Check sheet for the modelled part. Datum: model origin and axes. Units: mm. Face numbers are marked on the shaded views. A direction names the side the tool comes from. Give positions to 0.01 mm unless a question says otherwise; leave off trailing zeros. Order: outer loops, then holes, each group sorted by start corner. A loop starts at its lowest first (then second) coordinate and runs counter-clockwise, first axis right, second up.
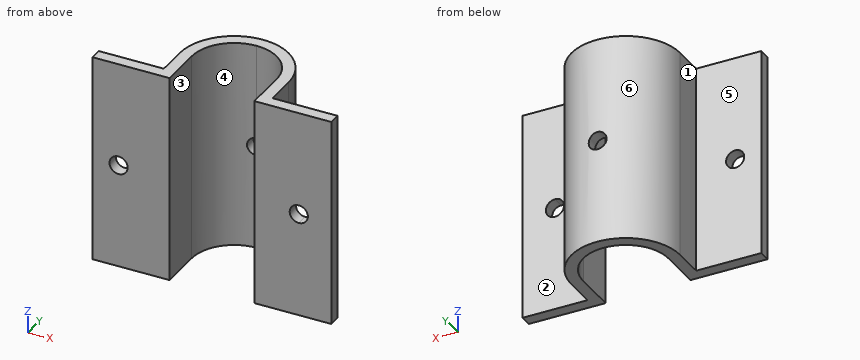
```python
from build123d import *

# Parameters (mm, degrees)
BOSS_EXTRUDE1_DEPTH = 70
SKETCH2_R           = 3.048
CUT_EXTRUDE1_DEPTH  = 70
FILLET1_R           = 14.224
FILLET2_RADIUS      = 18.224
FILLET2_LENGTH      = 70
SKETCH3_R           = 3
CUT_EXTRUDE2_DEPTH  = 70


with BuildPart() as part:
    # Sketch1 → Boss-Extrude1 (new body)
    with BuildSketch(Plane.XY):
        Polygon((-40.068, 0), (-18.224, 0), (-18.224, 28.448), (18.224, 28.448), (18.224, 0), (40.068, 0), (40.068, -4), (14.224, -4), (14.224, 24.448), (-14.224, 24.448), (-14.224, -4), (-40.068, -4), align=None)
    extrude(amount=BOSS_EXTRUDE1_DEPTH)

    # Sketch2 → Cut-Extrude1 (cut)
    with BuildSketch(Plane(origin=(0, 0, 0), x_dir=(1, 0, 0), z_dir=(0, 1, 0))):
        with Locations(Location((-31.280253866, -35, 0), (0, 0, 180))):
            Circle(SKETCH2_R)
        with BuildLine():
            ThreePointArc((32.194, -35), (31.301261469, -32.844738531), (29.146, -31.952))
            Line((29.146, -31.952), (29.146, -38.048))
            ThreePointArc((29.146, -38.048), (31.301261469, -37.155261469), (32.194, -35))
        make_face()
        with BuildLine():
            Line((29.146, -38.048), (29.146, -31.952))
            ThreePointArc((29.146, -31.952), (26.098, -35), (29.146, -38.048))
        make_face()
    extrude(amount=-CUT_EXTRUDE1_DEPTH, mode=Mode.SUBTRACT)

    # Fillet1
    fillet1_edges = [part.edges().sort_by_distance(p)[0] for p in [
        (14.224, 24.448, 35),
        (-14.224, 24.448, 35),
    ]]
    fillet(fillet1_edges, radius=FILLET1_R - 0.0001)  # a hair under: the kernel refuses the full size

    # Fillet2: full round fillet: the end face becomes a half cylinder, R = half its width
    fillet2_face = Plane((0, 28.448, 35), x_dir=(0, 0, 1), z_dir=(0, 1, 0))  # on the end face: x along it, z out of the body
    fillet2_slab = fillet2_face.offset(-FILLET2_RADIUS / 2) * Box(FILLET2_LENGTH, 2 * FILLET2_RADIUS, FILLET2_RADIUS, mode=Mode.PRIVATE)  # the body's end, R deep
    fillet2_round = Plane((0, 10.224, 35), x_dir=(0, 1, 0), z_dir=(0, 0, 1)) * Cylinder(FILLET2_RADIUS, FILLET2_LENGTH, mode=Mode.PRIVATE)  # its axis R under the face
    add(fillet2_slab - fillet2_round, mode=Mode.SUBTRACT)

    # Sketch3 → Cut-Extrude2 (cut)
    with BuildSketch(Plane(origin=(0, 0, 0), x_dir=(1, 0, 0), z_dir=(0, 1, 0))):
        with Locations(Location((0, -35, 0), (0, 0, 90))):
            Circle(SKETCH3_R)
    extrude(amount=CUT_EXTRUDE2_DEPTH, mode=Mode.SUBTRACT)


solid = part.part
```
(1) Cross-section at C-C on z = 33.5. Enter the section's corners in (x, y), then the cut area to 3 significant figures.
Response values:
outline: (-40.07, -4) - (-33.93, -4) - (-33.93, 0) - (-40.07, 0) - close; (-28.63, -4) - (-14.22, -4) - (-14.22, 10.22) arc R14.22 cw to (-2.6, 24.21) - (-2.6, 28.26) arc R18.22 ccw to (-18.22, 10.22) - (-18.22, 0) - (-28.63, 0) - close; (2.6, 24.21) arc R14.22 cw to (14.22, 10.22) - (14.22, -4) - (26.49, -4) - (26.49, 0) - (18.22, 0) - (18.22, 10.22) arc R18.22 ccw to (2.6, 28.26) - close; (31.8, -4) - (40.07, -4) - (40.07, 0) - (31.8, 0) - close
area: 429 mm2
(2) Set-up check for the marked faces 1, 2 and 3: record each of +Z, -Z, +X, -X, +Y, -Y from which the full face is reachable in a straight line by a thin tool's end or side.
Response values:
face 1: +Z, -Z, -X, +Y
face 2: +Z, -Z, +X, +Y
face 3: +Z, -Z, -Y
(3) Gauge pin test, flat ends, axial feed: pin 1 Ø1.5 at (x, z) = (-10, 50.5) entering from -Y; pin 2 Ø8 at (y, z) = (10, 58.5) entering from -X; pin 3 Ø1 at (x, z) = (30.5, 19.5) entering from +Y. Record the tip position at first contact, or that the pin passes through.
Response values:
pin 1: stops at y = 19.54
pin 2: stops at x = -18.22
pin 3: stops at y = 0
(4) Material ranges on L1, parallel to X at y = 8, z = 48; L2, parallel to Y at x = -29, z = 53; L3, parallel to X at y = 17.5, z = 65, recorded low to high.
Response values:
L1: x = -18.22 to -14.22, 14.22 to 18.22
L2: y = -4 to 0
L3: x = -16.71 to -12.22, 12.22 to 16.71
(5) Cross-section at B-B on y = 8. Enter the section's corners in (x, z).
Response values:
outline: (-18.22, 0) - (-14.22, 0) - (-14.22, 70) - (-18.22, 70) - close; (14.22, 0) - (18.22, 0) - (18.22, 70) - (14.22, 70) - close
(6) Release check for a two-part mould opening along X. For the marked faces 4, 5 and 6 record: released by +X, released by -X, zero draft, split by the parting line, or undercut.
Response values:
face 4: undercut
face 5: zero draft
face 6: split by the parting line
(7) Cross-section at A-A on y = -1. Enter the section's corners in (x, z), then the cut area to 3 significant figures.
Response values:
outline: (-40.07, 0) - (-14.22, 0) - (-14.22, 70) - (-40.07, 70) - close; (14.22, 0) - (40.07, 0) - (40.07, 70) - (14.22, 70) - close; hole circle Ø6.1 at (-31.28, 35); hole circle Ø6.1 at (29.15, 35)
area: 3,560 mm2
(8) Cross-section at D-D on x = 30.5. Enter the section's corners in (y, z).
Response values:
outline: (-4, 0) - (0, 0) - (0, 32.27) - (-4, 32.27) - close; (-4, 37.73) - (0, 37.73) - (0, 70) - (-4, 70) - close
